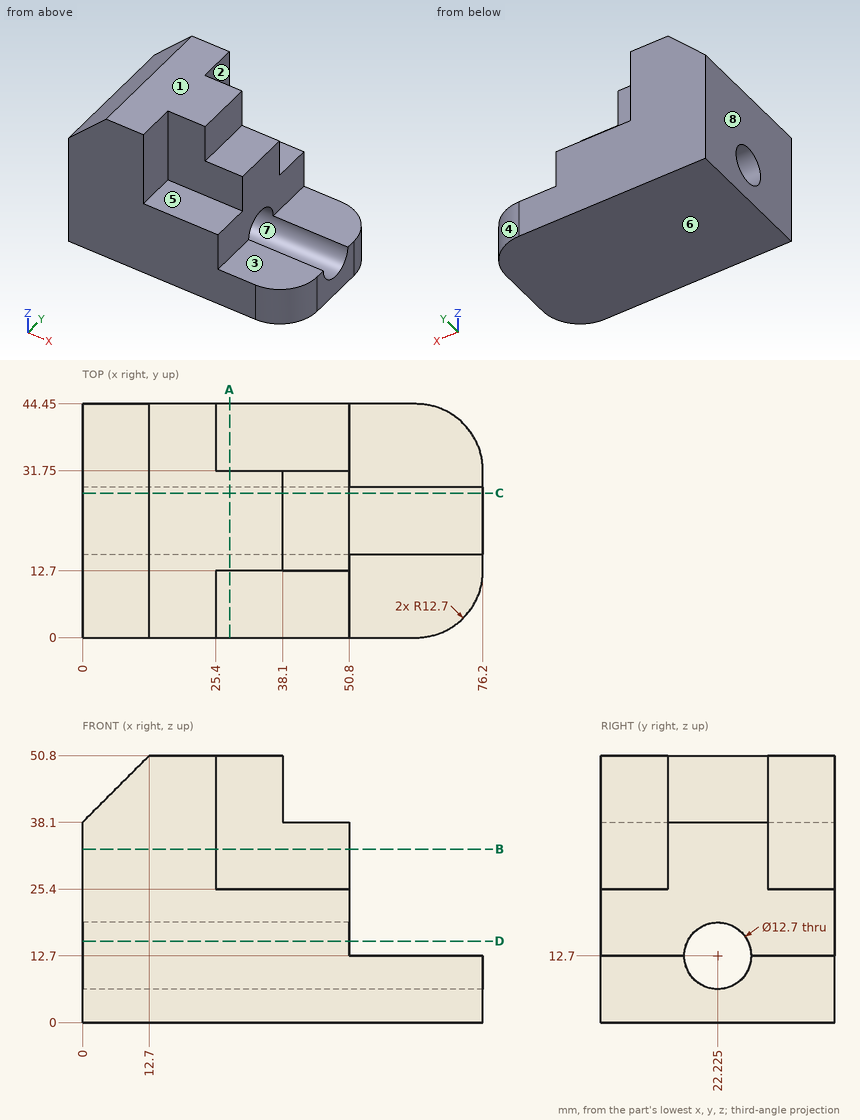
Study the drawing (mm; zero at the part's minimum x, y, z) and answer. A direction names the side the tool comes from. Round coordinates to 2 decimals unless told otherwise and drop trailing zeros. Loops run counter-clockwise (first coordinate to the right, second up) from the corner with the lowest first, then second, coordinate; pieces in that order, holes last.
Q1. Section A-A, the plane x = 28 is taken. Determine the outline of the cut face in (y, z) (3 decimals), then the cut area to 3 significant figures.
Q2. Section D-D, the plane z = 15.5 is taken. Determine the outline of the cut face in (x, y), then the cut area to 3 significant figures.
Q3. Find the intervals of material crossed by line 1 (Y direction, x = 32, z = 12.7) (3 decimals); line 2 (X direction, y = 22.5, z = 23); line 3 (X direction, y = 34, z = 27), in increasing order.
Q4. Section C-C, the plane y = 27.5 is taken. Determine the outline of the cut face in (x, z), then the cut area to 3 significant figures.
Q5. Section B-B, the plane z = 33 is taken. Determine the outline of the cut face in (x, y), then the cut area to 3 significant figures.
Q6. For a pull along Z with two mould halves and no side action, classify the marked faces 6, 7 and 8 as released by +Z, released by -Z, zero draft, split by the parting line, or undercut.
Q7. Which of the six approach directions +Z, -Z, +X, -X, +Y, -Y give full straight-line access (tool end or side, diameter ignored) to the marked faces 1, 2, 3, 4 and 5?
Q8. Given pin 1 Ø14 at (y, z) = (36.5, 35) entering from +X; pin 2 Ø6.5 at (x, y) = (32, 8) entering from +Z; pin 3 Ø5 at (x, y) = (69.5, 36) entering from +Z, each flat-ended and moving along its own axis, determine where each tip first touches the part or whether it passes through.
Completed:
1. outline: (0, 0) - (44.45, 0) - (44.45, 25.4) - (31.75, 25.4) - (31.75, 50.8) - (12.7, 50.8) - (12.7, 25.4) - (0, 25.4) - close; hole circle Ø12.7 at (22.225, 12.7)
1. area: 1,490 mm2
2. outline: (0, 0) - (50.8, 0) - (50.8, 16.53) - (0, 16.53) - close; (0, 27.92) - (50.8, 27.92) - (50.8, 44.45) - (0, 44.45) - close
2. area: 1,680 mm2
3. line 1: y = 0 to 15.875, 28.575 to 44.45
3. line 2: x = 0 to 50.8
3. line 3: x = 0 to 25.4
4. outline: (0, 0) - (76.2, 0) - (76.2, 9.16) - (0, 9.16) - close; (0, 16.24) - (50.8, 16.24) - (50.8, 38.1) - (38.1, 38.1) - (38.1, 50.8) - (12.7, 50.8) - (0, 38.1) - close
4. area: 2,210 mm2
5. outline: (0, 0) - (25.4, 0) - (25.4, 12.7) - (50.8, 12.7) - (50.8, 31.75) - (25.4, 31.75) - (25.4, 44.45) - (0, 44.45) - close
5. area: 1,610 mm2
6. face 6: released by -Z
6. face 7: undercut
6. face 8: zero draft
7. face 1: +Z, +X, -X, +Y, -Y
7. face 2: +Z, +X, +Y
7. face 3: +Z, +X, +Y, -Y
7. face 4: +Z, -Z, +X, +Y
7. face 5: +Z, +X, -Y
8. pin 1: stops at x = 50.8
8. pin 2: stops at z = 25.4
8. pin 3: stops at z = 12.7
